Geometry: final body of the model. Coordinates: model frame, mm. A direction names the side the tool comes from. Coordinates: 2 decimals unless noted, no trailing zeros. Loops run counter-clockwise (first coordinate to the right, second up) from the corner with the lowest first, then second, coordinate; pieces in that order, holes last. Notation, with made-up numbers: M -1.5,1.5 L 33.5,1.5 A10 ccw 33.5,5.5 Z; hole C 14,-21 d3. An arc over 180 degrees is marked long. Write each question's results on one line, items separated by ' | '. Start each with the question number.
Autodesk Inventor part; units mm, degrees
ref_plane "YZ Plane" through (0, 0, 0) normal (1, 0, 0) x (0, 1, 0)
ref_plane "XZ Plane" through (0, 0, 0) normal (0, 1, 0) x (-1, 0, 0)
ref_plane "XY Plane" through (0, 0, 0) normal (0, 0, 1) x (1, 0, 0)
sketch "Sketch1" plane through (0, 0, 0) normal (0, 0, 1) x (1, 0, 0)
  line L0 (-167.701, 0) -> (65.3284, 0)
  line L1 (76.0929, 0) -> (65.3284, 0)
  ellipse E0 centre (76.0929, 10) end of major axis (76.0929, 20) minor radius 7.0711 (76.0929, 0) -> (83.164, 10) ccw
  line L2 (83.164, 290) -> (83.164, 10)
  ellipse E1 centre (76.0929, 290) end of major axis (76.0929, 280) minor radius 7.0711 (83.164, 290) -> (76.0929, 300) ccw
  line L3 (65.3284, 300) -> (76.0929, 300)
  line L4 (65.3284, 300) -> (-167.701, 300)
  line L5 (-181.8431, 290) -> (-181.8431, 10)
  ellipse E2 centre (-167.701, 10) end of major axis (-181.8431, 10) minor radius 10 (-181.8431, 10) -> (-167.701, 0) ccw
  ellipse E3 centre (-167.701, 290) end of major axis (-153.5589, 290) minor radius 10 (-167.701, 300) -> (-181.8431, 290) ccw
  line L6 (65.3284, 300) -> (65.3284, 0)
  point P0 (0, 0)
extrude "Extrusion1" add sketch "Sketch1" against normal blind 1 contours E2 L5 E3 L4 L6 L0
ref_plane "Work Plane1" through (-51.1863, 0, 116.5147) normal (-0.7071, 0, -0.7071) x (-0.7071, 0, 0.7071)
sketch "Sketch2" plane through (-51.1863, 0, 116.5147) normal (-0.7071, 0, -0.7071) x (-0.7071, 0, 0.7071)
  line L0 (-164.7767, 0) -> (-164.7767, 300)
  line L1 (-190, 290) -> (-190, 10)
  arc A0 (-190, 10) -> (-180, 0) centre (-180, 10) ccw
  line L2 (-180, 0) -> (-164.7767, 0)
  line L3 (-164.7767, 300) -> (-180, 300)
  arc A1 (-180, 300) -> (-190, 290) centre (-180, 290) ccw
  point P0 (-118.5825, 0)
extrude "Extrusion2" add sketch "Sketch2" along normal blind 1
properties part number "Top Cover" material "Aluminum 6061"
Item 1: Set-up query: faces 1 (the flat face through (-60, 152, 0)), 2 (the flat face through (-60, 152, -1)). Return all of +Z, -Z, +X, -X, +Y, -Y with unobstructed straight access to the full face (end or side cutting, diameter ignored); none if empty.
Item 2: Section B-B, the plane x = -64. Return loops of the section in (y, z).
Item 3: Section C-C, the plane z = -5. Return loops of the section in (x, y), plus the area to 3 significant figures.
Item 4: Ray query, L1, parallel to Z at x = -9, y = 106.5; L2, parallel to X at y = 157, z = -8.25; L3, parallel to X at y = 286, z = -2.5. Return the intervals inside material, ascending. Write a range as [from, to].
Item 5: Contact query for flat-ended pins moving along their axis: P1, Ø5, axis at y = 160, z = -5.5, coming from the -X side; P2, Ø1.5, axis at y = 49, z = -15, coming from the +X side; P3, Ø4, axis at y = 245.5, z = -16, coming from the -X side. Output: stop coordinate, or through.
Solutions:
1) face 1: +Z, +X, -X, +Y, -Y | face 2: -Z, -X, +Y, -Y
2) outline: M 0,-1 L 300,-1 L 300,0 L 0,0 Z
3) outline: M 68.91,0 L 70.33,0 L 70.33,300 L 68.91,300 Z | area: 424 mm²
4) L1: z = [-1, 0] | L2: x = [72.16, 73.58] | L3: x = [66.41, 67.83]
5) P1: stops at x = 66.91 | P2: stops at x = 81.08 | P3: stops at x = 77.91
